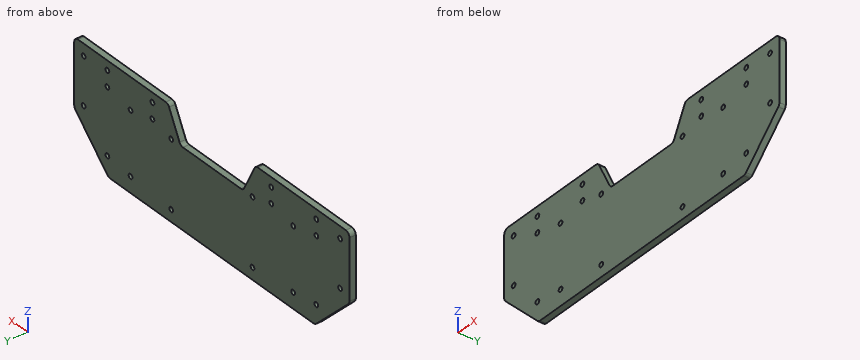
```python
from build123d import *

# Parameters (mm, degrees)
EXTRUDE_1_DEPTH     = 4
SKETCH_2_R          = 1.5
CUT_EXTRUDE_1_DEPTH = 4
SKETCH_3_W          = 10
SKETCH_3_H          = 69.678883607
SKETCH_3_H_2        = 93.047687854
CUT_EXTRUDE_2_DEPTH = 4
CUT_EXTRUDE_3_DEPTH = 4
EXTRUDE_2_DEPTH     = 4
SKETCH_6_R          = 1.5
CUT_EXTRUDE_4_DEPTH = 10
FILLET_1_R          = 3
SKETCH_7_R          = 1.503168948
SKETCH_7_R_2        = 1.5
CUT_EXTRUDE_5_DEPTH = 10
SKETCH_8_R          = 1.5
CUT_EXTRUDE_6_DEPTH = 10


with BuildPart() as part:
    # 草图1 → 凸台-拉伸1 (new body)
    with BuildSketch(Plane(origin=(0, 0, 0), x_dir=(1, 0, 0), z_dir=(0, 1, 0))):
        Polygon((-137.5, -35), (-67.5, -35), (-57.5, -35), (-47.5, -15), (2.5, -15), (12.5, -35), (22.5, -35), (92.5, -35), (92.5, 15), (72.5, 35), (-117.5, 35), (-137.5, 15), align=None)
    extrude(amount=EXTRUDE_1_DEPTH)

    # 草图2 → 切除-拉伸1 (cut)
    with BuildSketch(Plane(origin=(0, 4, 0), x_dir=(1, 0, 0), z_dir=(0, 1, 0))):
        with Locations(Location((-87.5, -15, 0), (0, 0, 270))):
            Circle(SKETCH_2_R)
        with Locations(Location((-87.5, 25, 0), (0, 0, 270))):
            Circle(SKETCH_2_R)
        with Locations(Location((42.5, 25, 0), (0, 0, 90))):
            Circle(SKETCH_2_R)
        with Locations(Location((42.5, -15, 0), (0, 0, 90))):
            Circle(SKETCH_2_R)
    extrude(amount=-CUT_EXTRUDE_1_DEPTH, mode=Mode.SUBTRACT)

    # 草图3 → 切除-拉伸2 (cut)
    with BuildSketch(Plane(origin=(0, 4, 0), x_dir=(1, 0, 0), z_dir=(0, 1, 0))):
        with Locations((-132.5, -0.160558196)):
            Rectangle(SKETCH_3_W, SKETCH_3_H)
        with Locations((87.5, 11.523843927)):
            Rectangle(SKETCH_3_W, SKETCH_3_H_2)
    extrude(amount=-CUT_EXTRUDE_2_DEPTH, mode=Mode.SUBTRACT)

    # 草图4 → 切除-拉伸3 (cut)
    with BuildSketch(Plane(origin=(0, 4, 0), x_dir=(1, 0, 0), z_dir=(0, 1, 0))):
        Polygon((-127.5, 12.5), (-92.197077218, 47.802922782), (-150.178982695, 47.802922782), align=None)
        Polygon((82.5, 12.5), (37.005283765, 57.994716235), (96.544114713, 56.205234398), align=None)
    extrude(amount=-CUT_EXTRUDE_3_DEPTH, mode=Mode.SUBTRACT)

    # 草图5 → 凸台-拉伸2 (add)
    with BuildSketch(Plane(origin=(0, 4, 0), x_dir=(1, 0, 0), z_dir=(0, 1, 0))):
        Polygon((-127.5, 12.5), (-132.5, 7.5), (-132.5, -35), (-127.5, -35), align=None)
        Polygon((82.5, -35), (82.5, 12.5), (87.5, 7.5), (87.5, -35), align=None)
    extrude(amount=-EXTRUDE_2_DEPTH)

    # 草图6 → 切除-拉伸4 (cut)
    with BuildSketch(Plane(origin=(0, 4, 0), x_dir=(1, 0, 0), z_dir=(0, 1, 0))):
        with Locations(Location((61, -29, 0), (0, 0, 270))):
            Circle(SKETCH_6_R)
        with Locations(Location((61, -19, 0), (0, 0, 270))):
            Circle(SKETCH_6_R)
        with Locations(Location((25, -19, 0), (0, 0, 270))):
            Circle(SKETCH_6_R)
        with Locations(Location((25, -29, 0), (0, 0, 270))):
            Circle(SKETCH_6_R)
        with Locations(Location((-70, -29, 0), (0, 0, 90))):
            Circle(SKETCH_6_R)
        with Locations(Location((-70, -19, 0), (0, 0, 90))):
            Circle(SKETCH_6_R)
        with Locations(Location((-106, -19, 0), (0, 0, 90))):
            Circle(SKETCH_6_R)
        with Locations(Location((-106, -29, 0), (0, 0, 90))):
            Circle(SKETCH_6_R)
    extrude(amount=-CUT_EXTRUDE_4_DEPTH, mode=Mode.SUBTRACT)

    # 圆角1
    fillet_1_edges = [part.edges().sort_by_distance(p)[0] for p in [
        (60, 2, -35),
        (-132.5, 2, -7.5),
        (-132.5, 2, 35),
        (87.5, 2, -7.5),
        (87.5, 2, 35),
        (12.5, 2, 35),
        (2.5, 2, 15),
        (-47.5, 2, 15),
        (-57.5, 2, 35),
        (-105, 2, -35),
    ]]
    fillet(fillet_1_edges, radius=FILLET_1_R)

    # 草图7 → 切除-拉伸5 (cut)
    with BuildSketch(Plane(origin=(0, 4, 0), x_dir=(1, 0, 0), z_dir=(0, 1, 0))):
        with Locations(Location((80, -27.5, 0), (0, 0, 270))):
            Circle(SKETCH_7_R)
        with Locations(Location((80, 2.5, 0), (0, 0, 270))):
            Circle(SKETCH_7_R)
        with Locations(Location((-125, 2.5, 0), (0, 0, 90))):
            Circle(SKETCH_7_R)
        with Locations(Location((-125, -27.5, 0), (0, 0, 90))):
            Circle(SKETCH_7_R)
        with Locations(Location((10, -15, 0), (0, 0, 270))):
            Circle(SKETCH_7_R_2)
        with Locations(Location((10, 27.5, 0), (0, 0, 270))):
            Circle(SKETCH_7_R_2)
        with Locations(Location((-55, 27.5, 0), (0, 0, 90))):
            Circle(SKETCH_7_R_2)
        with Locations(Location((-55, -15, 0), (0, 0, 90))):
            Circle(SKETCH_7_R_2)
    extrude(amount=-CUT_EXTRUDE_5_DEPTH, mode=Mode.SUBTRACT)

    # 草图8 → 切除-拉伸6 (cut)
    with BuildSketch(Plane(origin=(0, 4, 0), x_dir=(1, 0, 0), z_dir=(0, 1, 0))):
        with Locations(Location((61, 22.5, 0), (0, 0, 270))):
            Circle(SKETCH_8_R)
        with Locations(Location((-106, 22.5, 0), (0, 0, 90))):
            Circle(SKETCH_8_R)
    extrude(amount=-CUT_EXTRUDE_6_DEPTH, mode=Mode.SUBTRACT)


solid = part.part
```
The listing builds one solid part. Answer for the finished solid, in the listing's coordinates (mm). Round coordinates to 2 decimals unless told otherwise and drop trailing zeros. Loops run counter-clockwise (first coordinate to the right, second up) from the corner with the lowest first, then second, coordinate; pieces in that order, holes last.
Q1. Find the intervals of material crossed by line 1 (Z direction, x = 42.5, y = 3.2); line 2 (X direction, y = 3.3, z = -2.5); line 3 (Z direction, x = -70, y = 2.7), in increasing order.
Q2. Section C-C, the plane x = 68.5 is taken. Determine the outline of the cut face in (y, z), then the cut area to 3 significant figures.
Q3. Given pin 1 Ø2 at (y, z) = (2.5, -8) entering from -X; pin 2 Ø2.5 at (x, z) = (42.5, -25) entering from +Y; pin 3 Ø4 at (x, z) = (61, -22.5) entering from -Y; pin 4 Ø1 at (y, z) = (3, -19.5) entering from -X, each flat-ended and moving along its own axis, determine where each tip first touches the part or whether it passes through.
Q4. Section A-A, the plane y = 1.3 is taken. Count the separate pieces of the cut face and the enclosed holes in it, then the cut area to 3 significant figures.
Q5. Section B-B, the plane z = -12 is taken. Determine the outline of the cut face in (x, y).
Completed:
1. line 1: z = -35 to -26.5, -23.5 to 13.5, 16.5 to 35
1. line 2: x = -132.5 to -126.5, -123.5 to 78.5, 81.5 to 87.5
1. line 3: z = -35 to 17.5, 20.5 to 27.5, 30.5 to 35
2. outline: (0, -26.5) - (4, -26.5) - (4, 35) - (0, 35) - close
2. area: 246 mm2
3. pin 1: stops at x = -132.41
3. pin 2: passes through
3. pin 3: stops at y = 0
3. pin 4: stops at x = -121
4. separate pieces: 1
4. enclosed holes: 22
4. area: 13,300 mm2
5. outline: (-128, 0) - (83, 0) - (83, 4) - (-128, 4) - close
